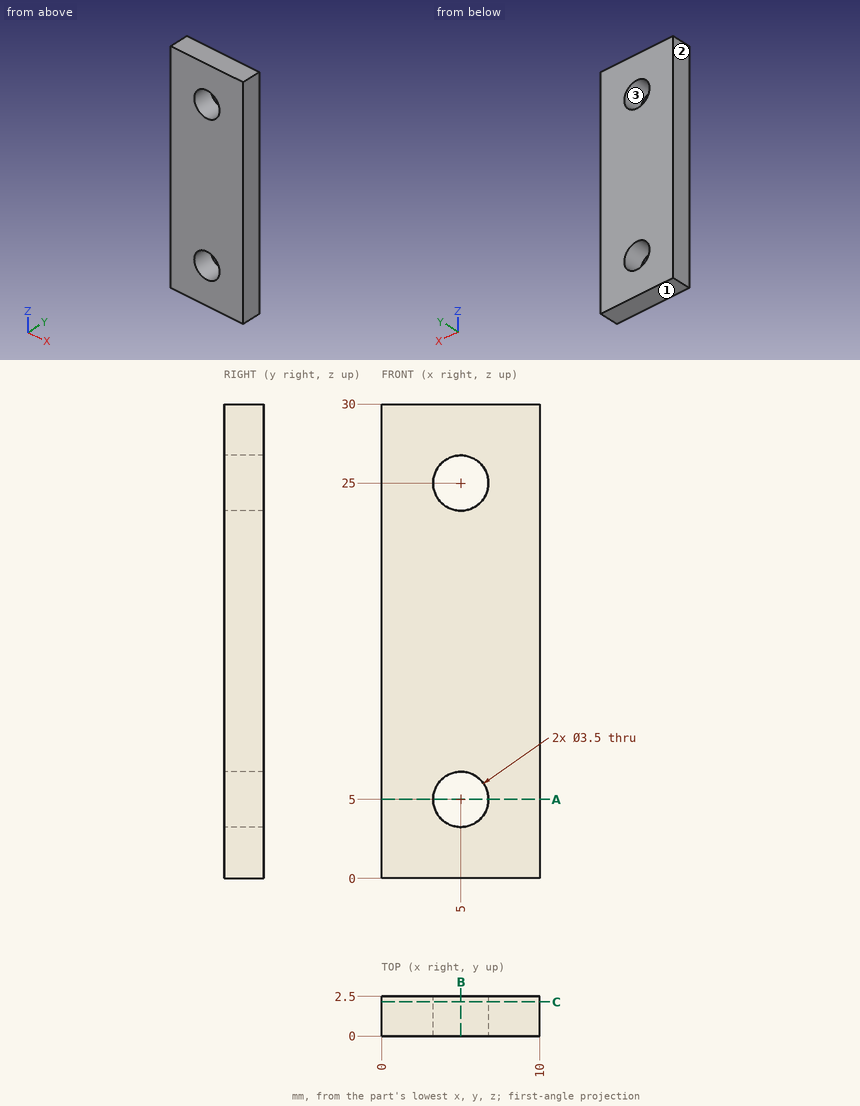
Part print with two shaded views. Sizes in mm from the minimum x, y, z corner. Coordinates: 2 decimals unless noted, no trailing zeros. Write each loop counter-clockwise with the first axis right and the second up, starting at its lowest first coordinate (ties: lowest second). Pieces come first, ordered by that corner, then holes. Notation, with made-up numbers: (47.25, 32) - (85.25, 32) arc R20 cw to (85.25, 59) - close; hole circle Ø3 at (-40, 25.5). An arc over 180 degrees is marked (long way). One line per item, written item: value. Start each with the question number.
1. Mould opens along Z. For the marked faces 1, 2 and 3 say: released by +Z, released by -Z, zero draft, split by the parting line, or undercut.
2. Slice it at B-B (x = 5). Write the cut outline in (y, z).
3. Slice it at A-A (z = 5). Write the cut outline in (x, y).
4. Slice it at C-C (y = 2.15). Write the cut outline in (x, z).
5. Probe line 1 (Z direction, x = 5, y = 2.1); line 2 (X direction, y = 1.05, z = 25); line 3 (Z direction, x = 6.25, y = 1.7). List the from-to ranges inside material, lowest first. Write a range as from..to.
Answers below:
1. face 1: released by -Z
1. face 2: zero draft
1. face 3: undercut
2. outline: (0, 0) - (2.5, 0) - (2.5, 3.25) - (0, 3.25) - close; (0, 6.75) - (2.5, 6.75) - (2.5, 23.25) - (0, 23.25) - close; (0, 26.75) - (2.5, 26.75) - (2.5, 30) - (0, 30) - close
3. outline: (0, 0) - (3.25, 0) - (3.25, 2.5) - (0, 2.5) - close; (6.75, 0) - (10, 0) - (10, 2.5) - (6.75, 2.5) - close
4. outline: (0, 0) - (10, 0) - (10, 30) - (0, 30) - close; hole circle Ø3.5 at (5, 5); hole circle Ø3.5 at (5, 25)
5. line 1: z = 0..3.25, 6.75..23.25, 26.75..30
5. line 2: x = 0..3.25, 6.75..10
5. line 3: z = 0..3.78, 6.22..23.78, 26.22..30
